Geometry: final body of the model. Coordinates: model frame, mm. A direction names the side the tool comes from. Give positions to 0.01 mm unless a question says otherwise; leave off trailing zeros. Order: outer loops, then holes, each group sorted by start corner. A loop starts at its lowest first (then second) coordinate and runs counter-clockwise, first axis right, second up. Notation, with made-up numbers: M -12.5,1.25 L -1.5,1.25 A36 ccw -1.5,35.25 Z; hole C 64.5,-8 d1. An arc over 180 degrees is marked long. Use CSV: the item, a comma, the result in double quotes.
```python
from build123d import *

# Parameters (mm, degrees)
F0_W     = 30
F0_H     = 25
F0_R     = 1.5
F0_R_2   = 1.8
F1_DEPTH = 8
F2_W     = 1.5
F2_H     = 3
F3_DEPTH = 8
F4_DEPTH = 5
F5_W     = 4.9
F5_H     = 2.8
F6_DEPTH = 3
F7_W     = 8
F7_H     = 8
F8_DEPTH = 5


with BuildPart() as f1:
    # F0 (on Front) → F1 (new body)
    with BuildSketch(Plane.XZ):
        with Locations((2.5, -2.5)):
            Rectangle(F0_W, F0_H)
        with Locations((-7.5, -10)):
            Circle(F0_R, mode=Mode.SUBTRACT)
        with Locations((2.5, -10)):
            Circle(F0_R, mode=Mode.SUBTRACT)
        with Locations((12.5, -10)):
            Circle(F0_R, mode=Mode.SUBTRACT)
        with Locations((-7.5, 5)):
            Circle(F0_R_2, mode=Mode.SUBTRACT)
        with Locations((12.5, 5)):
            Circle(F0_R_2, mode=Mode.SUBTRACT)
    extrude(amount=-F1_DEPTH)

    # F2 (on face) → F3 (join)
    with BuildSketch(Plane(origin=(0, 8, 0), x_dir=(-1, 0, 0), z_dir=(0, 1, 0))):
        Polygon((-17.5, -9), (-20.5, -9), (-20.5, -15), (-17.5, -15), (-17.5, -13.5), (-19, -13.5), (-19, -10.5), (-17.5, -10.5), align=None)
        Polygon((-17.5, 8.5), (-17.5, 10), (-20.5, 10), (-20.5, 4), (-17.5, 4), (-17.5, 5.5), (-19, 5.5), (-19, 8.5), align=None)
        Polygon((15.5, 10), (12.5, 10), (12.5, 8.5), (14, 8.5), (14, 5.5), (12.5, 5.5), (12.5, 4), (15.5, 4), align=None)
        Polygon((15.5, -15), (15.5, -9), (12.5, -9), (12.5, -10.5), (14, -10.5), (14, -13.5), (12.5, -13.5), (12.5, -15), align=None)
        with Locations((-18.25, 7)):
            Rectangle(F2_W, F2_H)
        with Locations((-18.25, -12)):
            Rectangle(F2_W, F2_H)
        with Locations((13.25, -12)):
            Rectangle(F2_W, F2_H)
        with Locations((13.25, 7)):
            Rectangle(F2_W, F2_H)
    extrude(amount=-F3_DEPTH)

    # F2 (on face) → F4 (cut)
    with BuildSketch(Plane(origin=(0, 8, 0), x_dir=(-1, 0, 0), z_dir=(0, 1, 0))):
        with Locations((-16.75, 7)):
            Rectangle(F2_W, F2_H)
        with Locations((-18.25, 7)):
            Rectangle(F2_W, F2_H)
        with Locations((-16.75, -12)):
            Rectangle(F2_W, F2_H)
        with Locations((-18.25, -12)):
            Rectangle(F2_W, F2_H)
        with Locations((13.25, -12)):
            Rectangle(F2_W, F2_H)
        with Locations((11.75, -12)):
            Rectangle(F2_W, F2_H)
        with Locations((13.25, 7)):
            Rectangle(F2_W, F2_H)
        with Locations((11.75, 7)):
            Rectangle(F2_W, F2_H)
    extrude(amount=-F4_DEPTH, mode=Mode.SUBTRACT)

    # F5 (on face) → F6 (join)
    with BuildSketch(Plane.YZ.offset(16)):
        Polygon((8.1, 8.4), (8, 8.4), (8, 5.6), (8.1, 5.6), (8.1, 4), (26.1, 4), (13.1, -9), (8.1, -9), (8.1, -10.6), (8, -10.6), (3.1, -10.6), (3.1, -13.4), (8, -13.4), (8.1, -13.4), (8.1, -13.5), (8.1, -15), (13.1, -15), (49.069655, -15), (55.997858, -15), (41.564102, 10), (38.1, 10), (8.1, 10), align=None)
        Polygon((34.585282, 4), (38.1, 4), (45.605553, -9), (21.585282, -9), align=None, mode=Mode.SUBTRACT)
        with Locations((5.55, 7)):
            Rectangle(F5_W, F5_H)
    extrude(amount=F6_DEPTH)

    # F7 (on face) → F8 (join)
    with BuildSketch(Plane(origin=(0, 35.503203, 20.497784), x_dir=(-1, 0, 0), z_dir=(0, 0.866025, 0.5))):
        with Locations((-23, -26.555553)):
            Rectangle(F7_W, F7_H)
        with Locations((-12, -26.555553)):
            Rectangle(F7_W, F7_H)
    extrude(amount=-F8_DEPTH)


solid = f1.part
```
1. Pin query (flat end, axial travel): pin 1 Ø1.5 at (y, z) = (6, -12.5) entering from +X; pin 2 Ø1.8 at (x, z) = (17, 4.5) entering from -Y; pin 3 Ø6.5 at (y, z) = (5.5, -4.5) entering from -X; pin 4 Ø1 at (y, z) = (20, -10) entering from +X. Return the tip coordinate at first contact, or that it passes through.
Answer:
pin 1,"x = 20.5"
pin 2,"y = 0"
pin 3,"x = -12.5"
pin 4,"x = 19"
2. Section D-D, the plane z = 2.25. Return the cut outline in (x, y), plus the area to 3 significant figures.
Answer:
outline,"M -12.5,0 L 17.5,0 L 17.5,8 L -12.5,8 Z; M 16,24.35 L 19,24.35 L 19,32.84 L 16,32.84 Z; M 16,39.11 L 19,39.11 L 19,46.04 L 16,46.04 Z"
area,"286 mm2"
3. Reachability of faces 1 (the face through (17.5, 19.7, -2.4)), 2 (the face through (23.056, 44.646, -0.268)), 3 (the face through (-11, 6, -12)) from +Z, -Z, +X, -X, +Y, -Y: full face, straight path, thin tool, end or side. Return the list, or none.
Answer:
face 1,"+X, -X"
face 2,"+Z, +X, -Y"
face 3,"+Y"
4. Section A-A, the plane x = 2.5. Return the cut outline in (y, z).
Answer:
outline,"M 0,-15 L 8,-15 L 8,-11.5 L 0,-11.5 Z; M 0,-8.5 L 8,-8.5 L 8,10 L 0,10 Z"
5. Line query: line 1 (Z direction, x = 12.5, y = 6.5); line 2 (Z direction, x = 12, y = 5); line 3 (X direction, y = 6.5, z = -12.5). Output: solid intervals per line, ascending.
Answer:
line 1,"-15 to -11.5, -8.5 to 3.2, 6.8 to 10"
line 2,"-15 to -11.41, -8.59 to 3.27, 6.73 to 10"
line 3,"-15.5 to -14, -11 to 20.5"
6. Pull-direction query (X, two-part tool) for faces 4 (the face through (-13, 6, 8.5)), 5 (the face through (17.48, 41.8, -2.41)), 6 (the face through (16, 26, -2)); classes: +X half, -X half, draft (parallel to the pull), parting line (faces both ways), or undercut.
Answer:
face 4,"undercut"
face 5,"draft"
face 6,"-X half"
7. Section C-C, the plane y = 19. Return the cut outline in (x, z), plus the area to 3 significant figures.
Answer:
outline,"M 16,-15 L 19,-15 L 19,-3.1 L 16,-3.1 Z; M 16,4 L 19,4 L 19,10 L 16,10 Z"
area,"53.7 mm2"
8. Section B-B, the plane x = 12.5. Return the cut outline in (y, z).
Answer:
outline,"M 0,-15 L 8,-15 L 8,-11.5 L 0,-11.5 Z; M 0,-8.5 L 8,-8.5 L 8,3.2 L 0,3.2 Z; M 0,6.8 L 8,6.8 L 8,10 L 0,10 Z; M 42.45,-1.54 L 46.45,-8.46 L 50.78,-5.96 L 46.78,0.96 Z"
